```python
from build123d import *

# Parameters (mm, degrees)
CROQUIS1_W              = 67
CROQUIS1_H              = 80
SALIENTE_EXTRUIR1_DEPTH = 17
CORTAR_EXTRUIR2_DEPTH   = 59.261822835
CROQUIS5_R              = 2.5
CORTAR_EXTRUIR3_DEPTH   = 59.261822835
REDONDEO1_R             = 2
REDONDEO2_R             = 3
REDONDEO3_R             = 5
CROQUIS6_W              = 8
CROQUIS6_H              = 14
CORTAR_EXTRUIR4_DEPTH   = 59.261822835


with BuildPart() as part:
    # Croquis1 → Saliente-Extruir1 (new body)
    with BuildSketch(Plane.XY):
        with Locations((5.3, 0)):
            Rectangle(CROQUIS1_W, CROQUIS1_H)
    extrude(amount=SALIENTE_EXTRUIR1_DEPTH)

    # Croquis4 → Cortar-Extruir2 (cut, through all)
    with BuildSketch(Plane.XY.offset(17)):
        Polygon((-28.2, 19.2), (-19.2, 19.2), (-19.2, 28.2), (19.2, 28.2), (19.2, 19.2), (28.2, 19.2), (28.2, -19.2), (19.2, -19.2), (19.2, -28.2), (-19.2, -28.2), (-19.2, -19.2), (-28.2, -19.2), align=None)
    extrude(amount=-CORTAR_EXTRUIR2_DEPTH, mode=Mode.SUBTRACT)

    # Croquis5 → Cortar-Extruir3 (cut, through all)
    with BuildSketch(Plane.XY.offset(17)):
        with Locations((-23.55, 23.55)):
            Circle(CROQUIS5_R)
        with Locations((23.55, 23.55)):
            Circle(CROQUIS5_R)
        with Locations((23.55, -23.55)):
            Circle(CROQUIS5_R)
        with Locations((-23.55, -23.55)):
            Circle(CROQUIS5_R)
        with BuildLine():
            Line((-23, 36.5), (-13, 36.5))
            ThreePointArc((-13, 36.5), (-10.5, 34), (-13, 31.5))
            Line((-13, 31.5), (-23, 31.5))
            ThreePointArc((-23, 31.5), (-25.5, 34), (-23, 36.5))
        make_face()
        with BuildLine():
            Line((13, 36.5), (23, 36.5))
            ThreePointArc((23, 36.5), (25.5, 34), (23, 31.5))
            Line((23, 31.5), (13, 31.5))
            ThreePointArc((13, 31.5), (10.5, 34), (13, 36.5))
        make_face()
        with BuildLine():
            Line((-23, -31.5), (-13, -31.5))
            ThreePointArc((-13, -31.5), (-10.5, -34), (-13, -36.5))
            Line((-13, -36.5), (-23, -36.5))
            ThreePointArc((-23, -36.5), (-25.5, -34), (-23, -31.5))
        make_face()
        with BuildLine():
            Line((13, -31.5), (23, -31.5))
            ThreePointArc((23, -31.5), (25.5, -34), (23, -36.5))
            Line((23, -36.5), (13, -36.5))
            ThreePointArc((13, -36.5), (10.5, -34), (13, -31.5))
        make_face()
    extrude(amount=-CORTAR_EXTRUIR3_DEPTH, mode=Mode.SUBTRACT)

    # Redondeo1
    redondeo1_edges = [part.edges().sort_by_distance(p)[0] for p in [
        (-19.2, 28.2, 8.5),
        (19.2, 28.2, 8.5),
        (28.2, 19.2, 8.5),
        (28.2, -19.2, 8.5),
        (19.2, -28.2, 8.5),
        (-19.2, -28.2, 8.5),
    ]]
    fillet(redondeo1_edges, radius=REDONDEO1_R)

    # Redondeo2
    redondeo2_edges = [part.edges().sort_by_distance(p)[0] for p in [
        (-19.2, 19.2, 8.5),
        (19.2, 19.2, 8.5),
        (19.2, -19.2, 8.5),
        (-19.2, -19.2, 8.5),
    ]]
    fillet(redondeo2_edges, radius=REDONDEO2_R)

    # Redondeo3
    redondeo3_edges = [part.edges().sort_by_distance(p)[0] for p in [
        (-28.2, 40, 8.5),
        (38.8, 40, 8.5),
        (38.8, -40, 8.5),
        (-28.2, -40, 8.5),
    ]]
    fillet(redondeo3_edges, radius=REDONDEO3_R)

    # Croquis6 → Cortar-Extruir4 (cut, through all)
    with BuildSketch(Plane.XY.offset(17)):
        with Locations((28.2, 0)):
            Rectangle(CROQUIS6_W, CROQUIS6_H)
    extrude(amount=-CORTAR_EXTRUIR4_DEPTH, mode=Mode.SUBTRACT)


solid = part.part
```
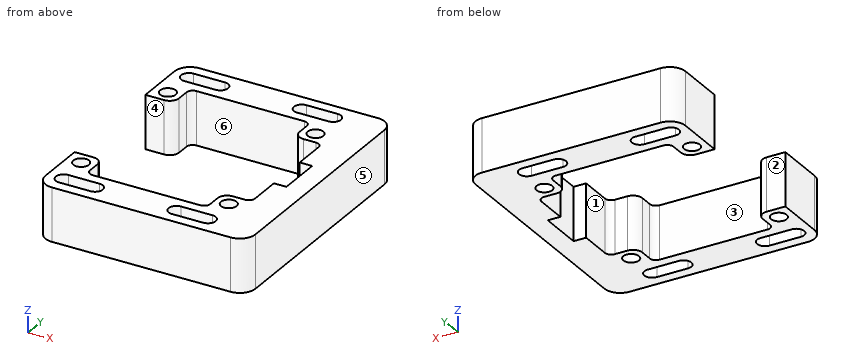
Can you work these out from the model? Positions are in its coordinate system, mm. Face numbers are marked on the shaded views. A direction names the side the tool comes from. Coordinates: 2 decimals unless noted, no trailing zeros. Loops run counter-clockwise (first coordinate to the right, second up) from the corner with the lowest first, then second, coordinate; pieces in that order, holes last. Notation, with made-up numbers: M 59,-35.75 L 75,-35.75 A20 cw 75,-0.75 Z; hole C 79,34 d6. An arc over 180 degrees is marked long. Put each result on its own line as item: value. Start each with the question number.
(1) Imagine slicing it at C-C on z = 9. Give the number of separate pieces and of enclosed holes in the cut face, and give its area (3 significant figures).
(2) Imagine slicing it at B-B on y = 23.55. List the corners of the cut face in (x, z) for me.
(3) I need wall thicknesses on probe 1 along Y at (x, z) = (-16.5, 10.75); probe 2 along Y at (x, z) = (-4, 7.75); probe 3 along Y at (x, z) = (-23.55, 5). Which ranges of each line are inside material? Lowest first, please.
(4) We'd pull the mould along X, two halves only. Please class the marked faces 1, 2 and 3: +X half, -X half, draft (parallel to the pull), parting line (faces both ways), or undercut.
(5) Will these pins go through, and if not, where does the flat tip stop? pin 1 Ø8 at (x, y) = (-23.55, 23.55) entering from -Z; pin 2 Ø3 at (x, z) = (-26.5, 9) entering from -Y; pin 3 Ø6 at (y, z) = (-6, 8.5) entering from -X; pin 4 Ø4 at (y, z) = (0.5, 5) entering from -X.
(6) Imagine slicing it at D-D on y = -8.5. List the corners of the cut face in (x, z) for me, and give its area (3 significant figures).
(7) Which directions (+Z, -Z, +X, -X, +Y, -Y) give clear straight access to the entire face, cutting with the end or side of a thin tool? Please do the marked faces 4, 5 and 6.
(8) Imagine slicing it at A-A on y = 34. List the corners of the cut face in (x, z) for me.
Worked answers:
1. separate pieces: 1
1. enclosed holes: 8
1. area: 2,070 mm2
2. outline: M -28.2,0 L -26.05,0 L -26.05,17 L -28.2,17 Z; M -21.05,0 L -19.2,0 L -19.2,17 L -21.05,17 Z; M 19.2,0 L 21.05,0 L 21.05,17 L 19.2,17 Z; M 26.05,0 L 38.8,0 L 38.8,17 L 26.05,17 Z
3. probe 1: y = -40 to -36.5, -31.5 to -28.2, 28.2 to 31.5, 36.5 to 40
3. probe 2: y = -40 to -28.2, 28.2 to 40
3. probe 3: y = -39.99 to -36.44, -31.56 to -26.05, -21.05 to -19.2, 19.2 to 21.05, 26.05 to 31.56, 36.44 to 39.99
4. face 1: -X half
4. face 2: draft
4. face 3: undercut
5. pin 1: stops at z = 0
5. pin 2: stops at y = -39.66
5. pin 3: stops at x = 28.2
5. pin 4: stops at x = 32.2
6. outline: M 28.2,0 L 38.8,0 L 38.8,17 L 28.2,17 Z
6. area: 180 mm2
7. face 4: +Z, -Z, -X
7. face 5: +Z, -Z, +X, +Y, -Y
7. face 6: +Z, -Z
8. outline: M -28.2,0 L -25.5,0 L -25.5,17 L -28.2,17 Z; M -10.5,0 L 10.5,0 L 10.5,17 L -10.5,17 Z; M 25.5,0 L 38.8,0 L 38.8,17 L 25.5,17 Z
